```python
from build123d import *

# Parameters (mm, degrees)
BOSS_EXTRUDE1_DEPTH = 9.525
SKETCH2_R           = 0.75
CUT_EXTRUDE1_DEPTH  = 1.5875
CUT_EXTRUDE2_DEPTH  = 2.54


with BuildPart() as part:
    # Sketch1 → Boss-Extrude1 (new body)
    with BuildSketch(Plane.XY):
        with BuildLine():
            Line((0, 0), (0, 8.3725))
            ThreePointArc((0, 8.3725), (0.743948776, 10.168551224), (2.54, 10.9125))
            Line((2.54, 10.9125), (15.24, 10.9125))
            Line((15.24, 10.9125), (15.24, 12.5))
            Line((15.24, 12.5), (2.54, 12.5))
            ThreePointArc((2.54, 12.5), (-0.378583239, 11.291083239), (-1.5875, 8.3725))
            Line((-1.5875, 8.3725), (-1.5875, 0))
            Line((-1.5875, 0), (0, 0))
        make_face()
    extrude(amount=BOSS_EXTRUDE1_DEPTH)

    # Sketch2 → Cut-Extrude1 (cut)
    with BuildSketch(Plane(origin=(0, 0, 0), x_dir=(0, 0, -1), z_dir=(1, 0, 0))):
        with Locations((-2.25, 6.277)):
            Circle(SKETCH2_R)
    extrude(amount=-CUT_EXTRUDE1_DEPTH, mode=Mode.SUBTRACT)

    # Sketch3 → Cut-Extrude2 (cut)
    with BuildSketch(Plane.XZ.offset(-10.9125)):
        with BuildLine():
            ThreePointArc((4.6609, 4.7625), (6.2484, 3.175), (7.8359, 4.7625))
            Line((7.8359, 4.7625), (4.6609, 4.7625))
        make_face()
        with BuildLine():
            Line((4.6609, 4.7625), (7.8359, 4.7625))
            ThreePointArc((7.8359, 4.7625), (6.2484, 6.35), (4.6609, 4.7625))
        make_face()
        with BuildLine():
            ThreePointArc((9.9441, 4.7625), (11.5316, 3.175), (13.1191, 4.7625))
            Line((13.1191, 4.7625), (9.9441, 4.7625))
        make_face()
        with BuildLine():
            Line((9.9441, 4.7625), (13.1191, 4.7625))
            ThreePointArc((13.1191, 4.7625), (11.5316, 6.35), (9.9441, 4.7625))
        make_face()
    extrude(amount=-CUT_EXTRUDE2_DEPTH, mode=Mode.SUBTRACT)


solid = part.part
```
Part model, mm, in its own coordinate system. A direction names the side the tool comes from. Round coordinates to 2 decimals unless told otherwise and drop trailing zeros. Loops run counter-clockwise (first coordinate to the right, second up) from the corner with the lowest first, then second, coordinate; pieces in that order, holes last. Notation, with made-up numbers: (-11.5, -8) -> (29.5, -8) arc R22 cw to (29.5, 5) -> close; hole circle Ø2 at (54.25, -39). An arc over 180 degrees is marked (long way). Use one line per item in the form item = value. Start each with the question number.
Item 1: Drill centre lines: line 1 along X through (y, z) = (11.75, 3.75); line 2 along X through (y, z) = (2.5, 7); line 3 along Y through (x, z) = (12.5, 9.25). Where is each one in solid material? Low to high.
Item 2: Band-saw the part on A-A (z = 2.25). List the corners of the cut face in (x, y) (1 decimal), plus the area to 3 significant figures.
Item 3: Tool access for faces 1 (the flat face through (15.24, 12, 5)), 2 (the flat face through (0, 4, 5)): list every direction of +Z, -Z, +X, -X, +Y, -Y with a clear straight run to the whole face (end or side of a thin tool).
Item 4: Band-saw the part on C-C (z = 6.75). List the corners of the cut face in (x, y) (1 decimal), plus the area to 3 significant figures.
Item 5: Two-plate mould, pull along Y, no slides. Class faces 3 (the cylindrical face through (-0.783, 5.545, 2.413)), 4 (the cylindrical face through (0.724, 10.149, 4.696)), 5 (the cylindrical face through (-0.35, 11.32, 4.7)), 6 (the flat face through (3.7, 11.4, 0)): released by +Y, released by -Y, zero draft, split by the parting line, or undercut.
Item 6: Band-saw the part on D-D (z = 4.5). List the corners of the cut face in (x, y) (1 decimal), plus the area to 3 significant figures.
Item 7: Drop flat-ended pins along their axis: pin 1 Ø5 at (y, z) = (7.5, 7) entering from +X; pin 2 Ø4 at (y, z) = (5.5, 4.5) entering from +X; pin 3 Ø1.5 at (x, z) = (12.5, 6) entering from -Y. Give the stop position or say it passes through.
Item 8: Band-saw the part on B-B (y = 6.5). List the corners of the cut face in (x, z) (1 decimal).
Data:
q1.line_1 = 0.17 to 5.03, 7.47 to 10.31, 12.75 to 15.24
q1.line_2 = -1.59 to 0
q1.line_3 = 10.91 to 12.5
q2.outline = (-1.6, 0) -> (0, 0) -> (0, 5.5) -> (-1.6, 5.5) -> close; (-1.6, 7) -> (0, 7) -> (0, 8.4) arc R2.5 cw to (2.5, 10.9) -> (15.2, 10.9) -> (15.2, 12.5) -> (2.5, 12.5) arc R4.1 ccw to (-1.6, 8.4) -> close
q2.area = 39.4 mm^2
q3.face_1 = +Z, -Z, +X, +Y, -Y
q3.face_2 = +Z, -Z, +X, -Y
q4.outline = (-1.6, 0) -> (0, 0) -> (0, 8.4) arc R2.5 cw to (2.5, 10.9) -> (15.2, 10.9) -> (15.2, 12.5) -> (2.5, 12.5) arc R4.1 ccw to (-1.6, 8.4) -> close
q4.area = 41.8 mm^2
q5.face_3 = undercut
q5.face_4 = released by -Y
q5.face_5 = released by +Y
q5.face_6 = zero draft
q6.outline = (-1.6, 0) -> (0, 0) -> (0, 8.4) arc R2.5 cw to (2.5, 10.9) -> (4.7, 10.9) -> (4.7, 12.5) -> (2.5, 12.5) arc R4.1 ccw to (-1.6, 8.4) -> close; (7.8, 10.9) -> (10, 10.9) -> (10, 12.5) -> (7.8, 12.5) -> close; (13.1, 10.9) -> (15.2, 10.9) -> (15.2, 12.5) -> (13.1, 12.5) -> close
q6.area = 31.8 mm^2
q7.pin_1 = 0.59
q7.pin_2 = 0
q7.pin_3 = 10.91
q8.outline = (-1.6, 0) -> (0, 0) -> (0, 1.5) -> (-1.6, 1.5) -> close; (-1.6, 3) -> (0, 3) -> (0, 9.5) -> (-1.6, 9.5) -> close
